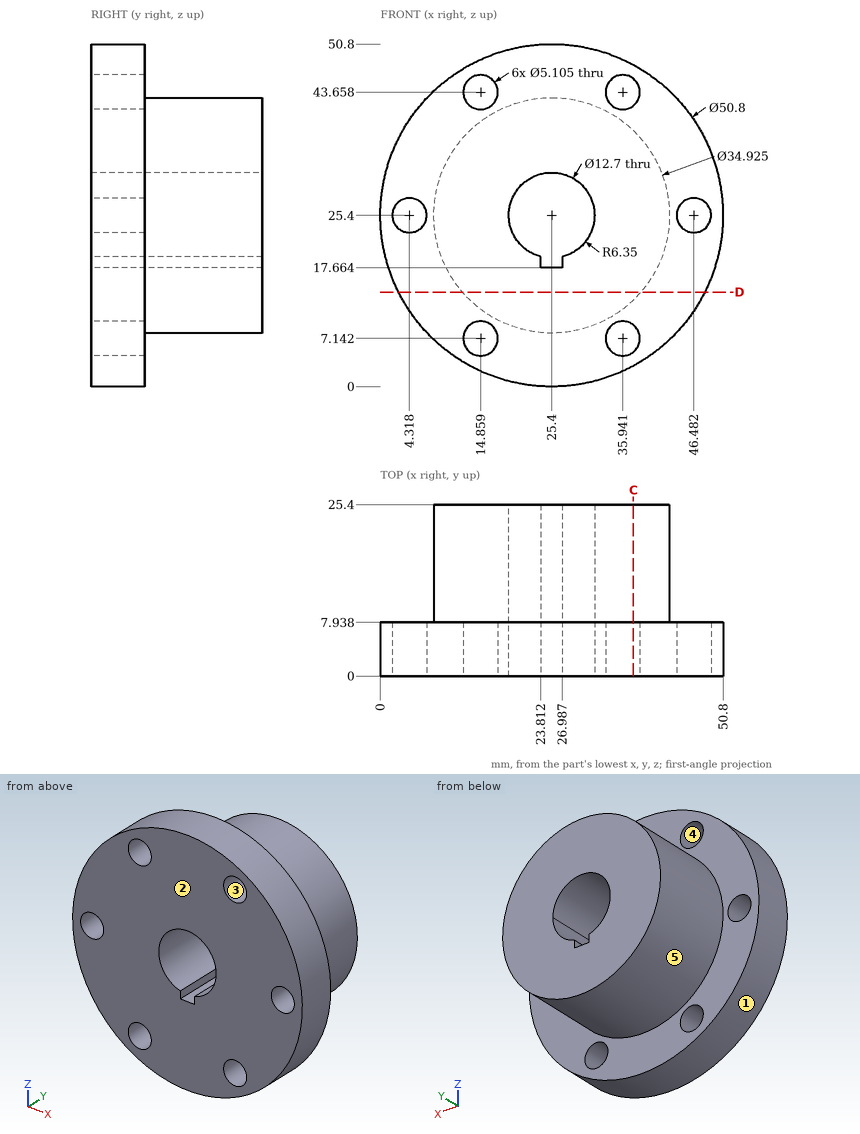
The drawing under review shows one solid part. Ordinate dimensions are in mm from its lowest x, y, z. A direction names the side the tool comes from. Round coordinates to 2 decimals unless told otherwise and drop trailing zeros. Order: outer loops, then holes, each group sorted by start corner. A loop starts at its lowest first (then second) coordinate and runs counter-clockwise, first axis right, second up. Notation, with made-up numbers: (-1, -14) -> (55, -14) arc R22 cw to (55, 9) -> close; hole circle Ø5 at (26, 52.5). An arc over 180 degrees is marked (long way). Return JSON: item names as keys, results as strings.
1. For the marked faces 4 and 5, list the 3-axis set-ups (+Z, -Z, +X, -X, +Y, -Y) from which the entire face can be reached by the end or side of a thin tool; tool diameter is ignored.
Answer block:
{"face 4": "+Y, -Y", "face 5": "+Y"}
2. Insertion check: P1, Ø6.5, axis at x = 14.86, z = 7.14, coming from the -Y side; P2, Ø5, axis at x = 11.5, y = 2.5, coming from the -Z side; P3, Ø12, axis at y = 3.5, z = 43, coming from the +X side; P4, Ø0.8, axis at y = 10.5, z = 18.5, coming from the +X side. Each pin has a flat end and moves straight along its axis. Give the tip position at first contact, or say it passes through.
Answer block:
{"P1": "stops at y = 0", "P2": "stops at z = 2.7", "P3": "stops at x = 48", "P4": "stops at x = 41.61"}
3. For L1, parallel to Z at x = 13, y = 7.5 (1 decimal); L2, parallel to X at y = 2.75, z = 43.5 (1 decimal); L3, parallel to X at y = 6, z = 5.5 (1 decimal), list the stretches that pass through material, from the lowest coordinate up. Write a range as [from, to].
Answer block:
{"L1": "z = [3.2, 5.4], [8.9, 41.9], [45.4, 47.6]", "L2": "x = [7.6, 12.3], [17.4, 33.4], [38.5, 43.2]", "L3": "x = [9.6, 12.9], [16.8, 34], [37.9, 41.2]"}
4. Take a section at D-D (z = 14). Write out the cut boundary in (x, y), then the cut area to 3 significant figures.
Answer block:
{"outline": "(2.7, 0) -> (48.1, 0) -> (48.1, 7.94) -> (38.63, 7.94) -> (38.63, 25.4) -> (12.17, 25.4) -> (12.17, 7.94) -> (2.7, 7.94) -> close", "area": "822 mm²"}
5. The part is to be moulded in two halves that separate along X. For the marked faces 1, 2 and 3, say which applies: +X half, -X half, draft (parallel to the pull), parting line (faces both ways), or undercut.
Answer block:
{"face 1": "parting line", "face 2": "draft", "face 3": "undercut"}
6. Take a section at C-C (x = 37.5). Write out the cut boundary in (y, z), then the cut area to 3 significant figures.
Answer block:
{"outline": "(0, 3.07) -> (7.94, 3.07) -> (7.94, 5.12) -> (0, 5.12) -> close; (0, 9.16) -> (7.94, 9.16) -> (7.94, 12.81) -> (25.4, 12.81) -> (25.4, 37.99) -> (7.94, 37.99) -> (7.94, 41.64) -> (0, 41.64) -> close; (0, 45.68) -> (7.94, 45.68) -> (7.94, 47.73) -> (0, 47.73) -> close", "area": "730 mm²"}
